Verification items for this drawing (mm, ordinates from the low corner). Coordinates: 2 decimals unless noted, no trailing zeros. Write each loop counter-clockwise with the first axis right and the second up, starting at its lowest first coordinate (ties: lowest second). Pieces come first, ordered by that corner, then holes. Notation, with made-up numbers: (-24, 49) -> (-1, 49) arc R24 cw to (-1, 77) -> close; hole circle Ø3 at (34, 28.25). An arc over 180 degrees is marked (long way). One line per question, with ' | ' between items.
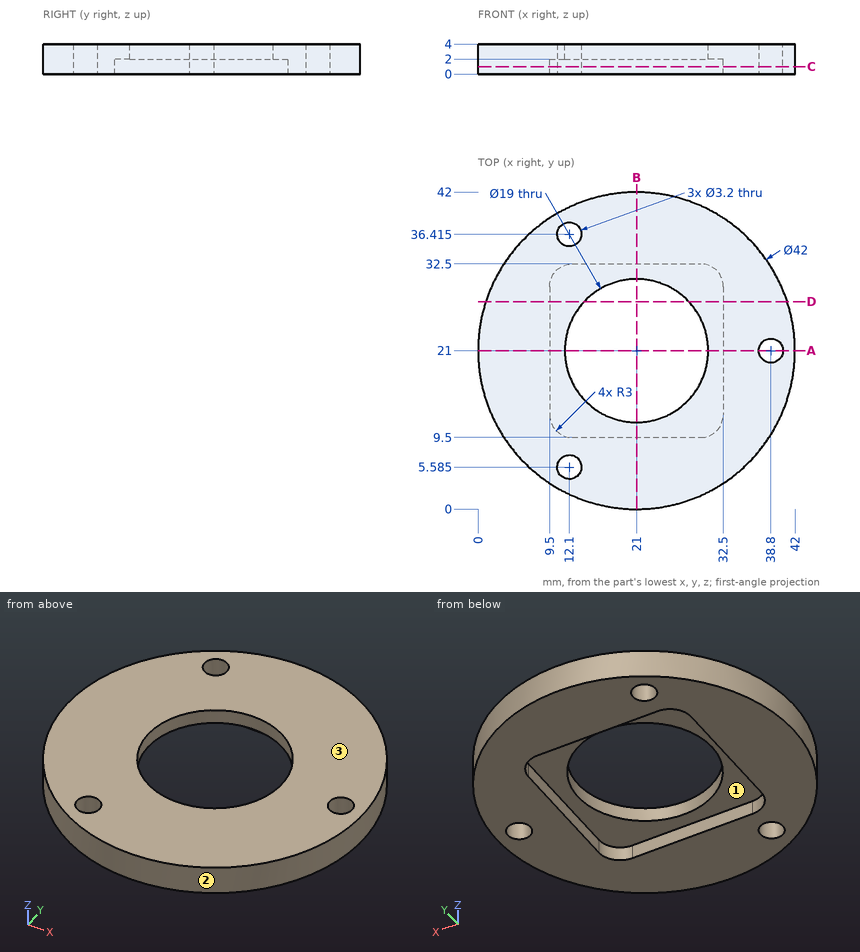
(1) Material ranges on line 1 (X direction, y = 21, z = 2.55); line 2 (X direction, y = 21, z = 1.1); line 3 (Y direction, x = 21, z = 2.5), recorded low to high.
Answers below:
line 1: x = 0 to 11.5, 30.5 to 37.2, 40.4 to 42 | line 2: x = 0 to 9.5, 32.5 to 37.2, 40.4 to 42 | line 3: y = 0 to 11.5, 30.5 to 42
(2) Cross-section at C-C (z = 1). Record the cut outline in (x, y) (1 decimal), plus the area to 3 significant figures.
Answers below:
outline: circle Ø42 at (21, 21); hole (9.5, 12.5) arc R3 ccw to (12.5, 9.5) -> (29.5, 9.5) arc R3 ccw to (32.5, 12.5) -> (32.5, 29.5) arc R3 ccw to (29.5, 32.5) -> (12.5, 32.5) arc R3 ccw to (9.5, 29.5) -> close; hole circle Ø3.2 at (12.1, 5.6); hole circle Ø3.2 at (12.1, 36.4); hole circle Ø3.2 at (38.8, 21) | area: 840 mm²
(3) Cross-section at D-D (y = 27.5). Record the cut outline in (x, z).
Answers below:
outline: (1.03, 0) -> (9.5, 0) -> (9.5, 2) -> (14.07, 2) -> (14.07, 4) -> (1.03, 4) -> close; (27.93, 2) -> (32.5, 2) -> (32.5, 0) -> (40.97, 0) -> (40.97, 4) -> (27.93, 4) -> close
(4) Cross-section at B-B (x = 21). Record the cut outline in (y, z), plus the area to 3 significant figures.
Answers below:
outline: (0, 0) -> (9.5, 0) -> (9.5, 2) -> (11.5, 2) -> (11.5, 4) -> (0, 4) -> close; (30.5, 2) -> (32.5, 2) -> (32.5, 0) -> (42, 0) -> (42, 4) -> (30.5, 4) -> close | area: 84.0 mm²
(5) Draft check along Y on the marked faces 1, 2 and 3. Enter one of: pulls with the +Y half, pulls with the -Y half, needs draft (parallel to the pull), parting line crosses it, or undercut.
Answers below:
face 1: undercut | face 2: parting line crosses it | face 3: needs draft
(6) Depth check by flat-ended pin: P1, Ø2.5, axis at x = 38.8, y = 21, coming from the +Z side; P2, Ø1.6, axis at x = 24.5, z = 0.5, coming from the +Y side; P3, Ø1.5, axis at x = 24.5, z = 1, coming from the -Y side; P4, Ø1.6, axis at y = 20, z = 1, coming from the +X side. Enter the tip coordinate at first touch or a pass-through.
Answers below:
P1: passes through | P2: stops at y = 41.83 | P3: stops at y = 0.18 | P4: stops at x = 42
(7) Cross-section at A-A (y = 21). Record the cut outline in (x, z), plus the area to 3 significant figures.
Answers below:
outline: (0, 0) -> (9.5, 0) -> (9.5, 2) -> (11.5, 2) -> (11.5, 4) -> (0, 4) -> close; (30.5, 2) -> (32.5, 2) -> (32.5, 0) -> (37.2, 0) -> (37.2, 4) -> (30.5, 4) -> close; (40.4, 0) -> (42, 0) -> (42, 4) -> (40.4, 4) -> close | area: 71.2 mm²
